Input: part model. Units: mm. Frame: model coordinates. A direction names the side the tool comes from. Coordinates: 2 decimals unless noted, no trailing zeros. Write each loop counter-clockwise with the first axis right and the second up, starting at its lowest first coordinate (ties: lowest second). Pieces come first, ordered by that corner, then holes.
1) Draft query along X for faces 4 (the flat face through (-11.073, 8, -5)), 5 (the flat face through (5, 15.875, -2)). Return one class per face: pulls with the +X half, pulls with the -X half, needs draft (parallel to the pull), parting line crosses it, or undercut.
2) Line query: L1, parallel to Y at x = 8, z = -2.2 (3 decimals); L2, parallel to Y at x = -16, z = 19 (3 decimals); L3, parallel to X at y = -2, z = 27. Output: solid intervals per line, ascending.
3) Section query A-A (y = 0). Output: boundary loops of the cut face in (x, z) (3 decimals), then the cut area to 3 significant figures.
4) Section query C-C (x = 8). Output: boundary loops of the cut face in (y, z) (3 decimals).
5) Set-up query: faces 1 (the flat face through (12.7, 4, 19)), 2 (the flat face through (8, -10.724, -5)), 3 (the flat face through (0, 0, -9.525)). Return all of +Z, -Z, +X, -X, +Y, -Y with unobstructed straight access to the full face (end or side cutting, diameter ignored); none if empty.
6) Section query D-D (y = -14). Output: boundary loops of the cut face in (x, z) (3 decimals).
7) Pin query (flat end, axial travel): pin 1 Ø8 at (x, z) = (-8, 23.5) entering from +Y; pin 2 Ø4 at (x, y) = (7, -11) entering from +Z. Return the tip coordinate at first contact, or that it passes through.
8) Section query B-B (z = 19.05). Output: boundary loops of the cut face in (x, y) (3 decimals).
from build123d import *

# Parameters (mm, degrees)
BOSS_EXTRUDE1_DEPTH     = 15.875
M2_5_CLEARANCE_HOLE1_D  = 3.1
F_1_4_CLEARANCE_HOLE1_D = 7.14248
SKETCH7_W               = 6.1468
SKETCH7_H               = 5.4483
CUT_EXTRUDE1_DEPTH      = 1.1771


with BuildPart() as part:
    # Sketch2 → Boss-Extrude1 (new body, symmetric)
    with BuildSketch(Plane(origin=(0, 0, 0), x_dir=(1, 0, 0), z_dir=(0, 1, 0))):
        Polygon((-12.7, 0), (-12.7, -38.1), (-19.05, -38.1), (-19.05, 9.525), (19.05, 9.525), (19.05, -38.1), (12.7, -38.1), (12.7, 0), align=None)
    extrude(amount=BOSS_EXTRUDE1_DEPTH, both=True)

    # M2.5 Clearance Hole1 (through all)
    with Locations(Plane(origin=(0, 0, -9.525), x_dir=(-1, 0, 0), z_dir=(0, 0, -1))):
        with Locations((8, 8), (-8, 8), (-8, -8), (8, -8)):
            Hole(M2_5_CLEARANCE_HOLE1_D / 2)

    # 1/4 Clearance Hole1 (through all)
    with Locations(Plane(origin=(19.05, 0, 0), x_dir=(0, 0, -1), z_dir=(1, 0, 0))):
        with Locations((-19.05, 0)):
            Hole(F_1_4_CLEARANCE_HOLE1_D / 2)

    # Sketch7 → Cut-Extrude1 (cut, symmetric)
    with BuildSketch(Plane.XY.offset(-4.7625)):
        with Locations((8, 8)):
            Rectangle(SKETCH7_W, SKETCH7_H)
        with Locations((-8, 8)):
            Rectangle(SKETCH7_W, SKETCH7_H)
        with Locations((-8, -8)):
            Rectangle(SKETCH7_W, SKETCH7_H)
        with Locations((8, -8)):
            Rectangle(SKETCH7_W, SKETCH7_H)
    extrude(amount=CUT_EXTRUDE1_DEPTH, both=True, mode=Mode.SUBTRACT)


solid = part.part
Answer:
1. face 4: undercut
1. face 5: needs draft
2. L1: y = -15.875 to -9.55, -6.45 to 6.45, 9.55 to 15.875
2. L2: y = -15.875 to -3.571, 3.571 to 15.875
2. L3: x = -19.05 to -12.7, 12.7 to 19.05
3. outline: (-19.05, -9.525) - (19.05, -9.525) - (19.05, 15.479) - (12.7, 15.479) - (12.7, 0) - (-12.7, 0) - (-12.7, 15.479) - (-19.05, 15.479) - close; (-19.05, 22.621) - (-12.7, 22.621) - (-12.7, 38.1) - (-19.05, 38.1) - close; (12.7, 22.621) - (19.05, 22.621) - (19.05, 38.1) - (12.7, 38.1) - close
3. area: 756 mm2
4. outline: (-15.875, -9.525) - (-9.55, -9.525) - (-9.55, -5.94) - (-10.724, -5.94) - (-10.724, -3.585) - (-9.55, -3.585) - (-9.55, 0) - (-15.875, 0) - close; (-6.45, -9.525) - (6.45, -9.525) - (6.45, -5.94) - (5.276, -5.94) - (5.276, -3.585) - (6.45, -3.585) - (6.45, 0) - (-6.45, 0) - (-6.45, -3.585) - (-5.276, -3.585) - (-5.276, -5.94) - (-6.45, -5.94) - close; (9.55, -9.525) - (15.875, -9.525) - (15.875, 0) - (9.55, 0) - (9.55, -3.585) - (10.724, -3.585) - (10.724, -5.94) - (9.55, -5.94) - close
5. face 1: +Z, +Y, -Y
5. face 2: none
5. face 3: -Z, +X, -X, +Y, -Y
6. outline: (-19.05, -9.525) - (19.05, -9.525) - (19.05, 38.1) - (12.7, 38.1) - (12.7, 0) - (-12.7, 0) - (-12.7, 38.1) - (-19.05, 38.1) - close
7. pin 1: passes through
7. pin 2: stops at z = 0
8. outline: (-19.05, -15.875) - (-12.7, -15.875) - (-12.7, -3.571) - (-19.05, -3.571) - close; (-19.05, 3.571) - (-12.7, 3.571) - (-12.7, 15.875) - (-19.05, 15.875) - close; (12.7, -15.875) - (19.05, -15.875) - (19.05, -3.571) - (12.7, -3.571) - close; (12.7, 3.571) - (19.05, 3.571) - (19.05, 15.875) - (12.7, 15.875) - close
